Source: three-view drawing plus pictorial views. Frame: mm from the lowest corner of the part. A direction names the side the tool comes from. Coordinates: 2 decimals unless noted, no trailing zeros. Write each loop counter-clockwise with the first axis right and the second up, starting at its lowest first coordinate (ties: lowest second). Pieces come first, ordered by that corner, then holes. Notation, with made-up numbers: (-37.5, 18) - (9.5, 18) arc R30 cw to (9.5, 54) - close; hole circle Ø2 at (66.25, 45.5). An arc over 180 degrees is marked (long way). Answer as a JSON object with one key per item and string values. Group by question number.
Item 1: First-contact query: pin 1 Ø4 at (y, z) = (43.5, 33.5) entering from -X (1 decimal); pin 2 Ø12 at (y, z) = (17.5, 35.5) entering from +X; pin 3 Ø2 at (y, z) = (34.5, 9.5) entering from +X (1 decimal); pin 4 Ø12 at (x, z) = (72, 16) entering from -Y. Flat tips, straight axial feed; report the tip coordinate or a pass-through.
Item 2: Line query: line 1 along Z through (x, y) = (68.5, 87) (1 decimal); line 2 along Y through (x, z) = (71, 66.5) (1 decimal); line 3 along X through (y, z) = (37, 64) (1 decimal). Output: solid intervals per line, ascending. Write a range as from..to.
Item 3: Set-up query: the marked faces 1 and 2. Return all of +Z, -Z, +X, -X, +Y, -Y with unobstructed straight access to the full face (end or side cutting, diameter ignored); none if empty.
Item 4: Section D-D on z = 80. Return loops of the section in (x, y) (1 decimal).
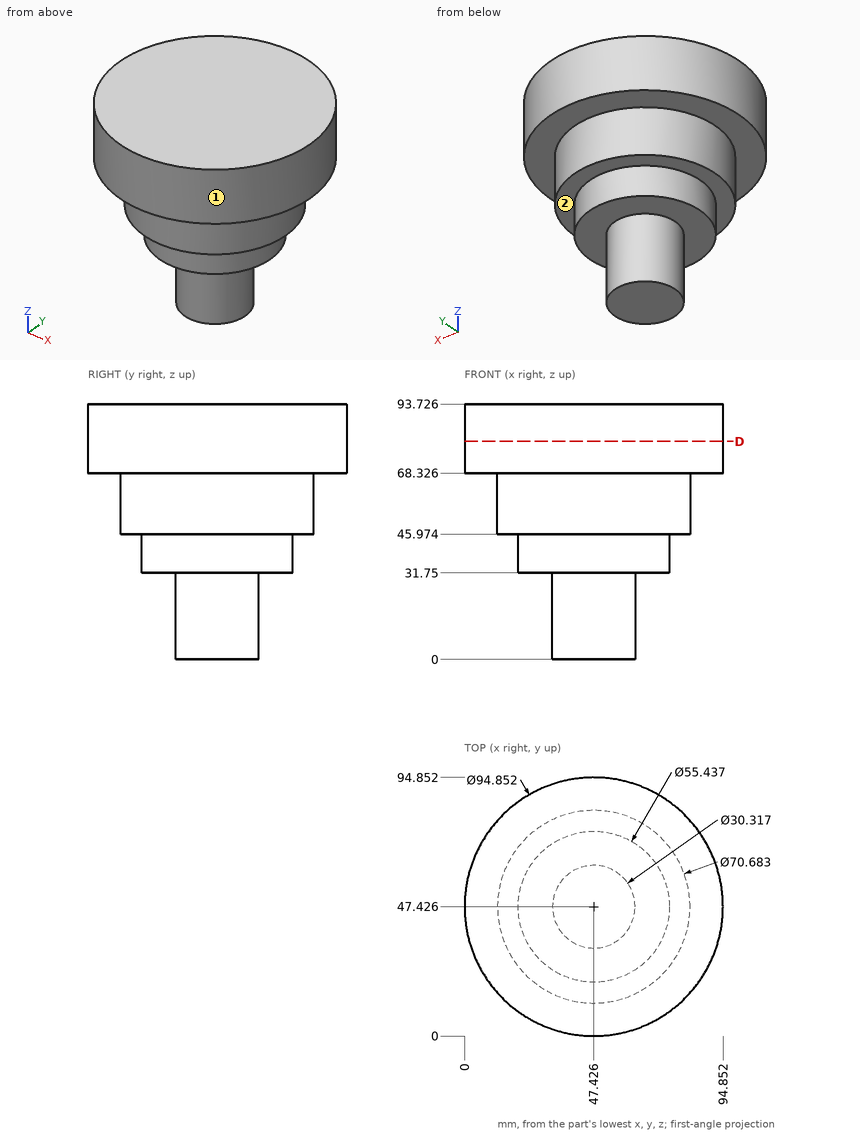
Checks:
{
 "1": {"pin 1": "x = 19.8", "pin 2": "x = 61.42", "pin 3": "x = 56.8", "pin 4": "through"},
 "2": {"line 1": "68.3..93.7", "line 2": "21.1..73.8", "line 3": "13.7..81.2"},
 "3": {"face 1": "+Z, -Z", "face 2": "-Z"},
 "4": {"outline": "circle Ø94.9 at (47.4, 47.4)"}
}
